Part model, mm, in its own coordinate system. A direction names the side the tool comes from. Give positions to 0.01 mm unless a question says otherwise; leave off trailing zeros. Write each loop counter-clockwise with the first axis right and the second up, starting at its lowest first coordinate (ties: lowest second). Pieces come first, ordered by that corner, then holes. Notation, with made-up numbers: M 9,-15.75 L 65,-15.75 A30 ccw 65,7.25 Z; hole C 26.25,59 d11. An arc over 180 degrees is marked long. Use CSV: the item, a comma, the result in double quotes. Start each with the question number.
Item 1: Which spindle directions (+Z, -Z, +X, -X, +Y, -Y) get a long thin tool onto all of the face, cutting with end or side? Do faces 5 (the flat face through (2, 2, 0)), 6 (the flat face through (81, 3, 8)). Say none if no direction does.
Item 2: Cut at A-A (z = 15). List the corners of the cut face in (x, y).
Item 3: Cut at B-B (y = 2.25). List the corners of the cut face in (x, z).
Item 4: Mould opens along X. For faces 1 (the flat face through (0, 3, 11)), 2 (the flat face through (3, 3, 9)), 3 (the flat face through (43, 3, 19)), 4 (the flat face through (84, 3, 11)) say: released by +X, released by -X, zero draft, split by the parting line, or undercut.
Item 5: Drill centre lines: line 1 (X direction, y = 1, z = 11.5); line 2 (X direction, y = 3, z = 16.75); line 3 (Z direction, x = 47.5, y = 3.5). Where is each one in solid material? Low to high. Write a range as [from, to].
Item 6: Pin check, flat tip, straight feed: pin 1 (5 mm diameter, centred on x = 73.5, z = 16, fed in from +Y). Stop position of the tip, or through.
Item 7: Cut at C-C (x = 63). List the corners of the cut face in (y, z), then the cut area to 3 significant figures.
from build123d import *


with BuildPart() as part:
    # По траектории1: sweep along a path in Эскиз1
    with BuildLine(Plane(origin=(0, 0, 0), x_dir=(1, 0, 0), z_dir=(0, 1, 0))) as sweep_1_path:
        Line((0, 0), (0, -22))
        Line((0, -22), (84, -22))
        Line((84, -22), (84, 0))
    # Эскиз2 → По траектории1 (sweep)
    with BuildSketch(Plane.XY):
        Polygon((6, 0), (0, 0), (0, 6), align=None)
    sweep(path=sweep_1_path.line, transition=Transition.RIGHT)


solid = part.part
Worked answers:
1,face 5,"-Z, +X, -X, +Y, -Y"
1,face 6,"-Z, +Y"
2,outline,"M 0,0 L 6,0 L 0,6 Z; M 78,0 L 84,0 L 84,6 Z"
3,outline,"M 0,0 L 3.75,0 L 3.75,18.25 L 80.25,18.25 L 80.25,0 L 84,0 L 84,22 L 0,22 Z"
4,face 1,"released by -X"
4,face 2,"undercut"
4,face 3,"undercut"
4,face 4,"released by +X"
5,line 1,"x = [0, 5], [79, 84]"
5,line 2,"x = [0, 3], [81, 84]"
5,line 3,"z = [19.5, 22]"
6,pin 1,"stops at y = 2.5"
7,outline,"M 0,16 L 6,22 L 0,22 Z"
7,area,"18.0 mm^2"
